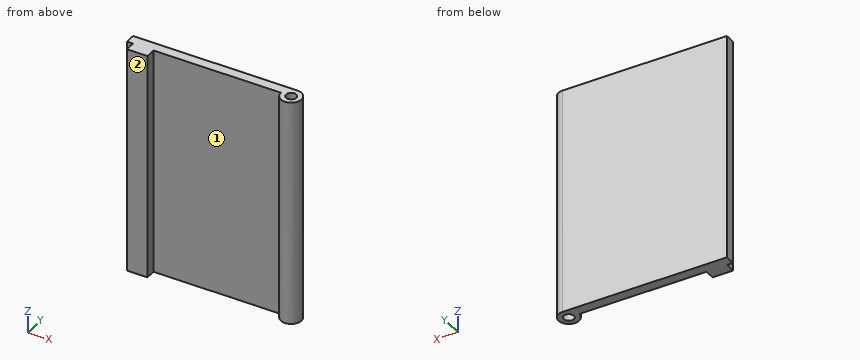
from build123d import *

# Parameters (mm, degrees)
F0_W     = 80
F0_H     = 110
F1_DEPTH = 5
F2_R     = 5
F2_W     = 10
F2_H     = 5
F3_DEPTH = 110
F4_R     = 2.5
F5_DEPTH = 110


with BuildPart() as f1:
    # F0 (on Front) → F1 (new body)
    with BuildSketch(Plane.XZ):
        with Locations((40, 55)):
            Rectangle(F0_W, F0_H)
    extrude(amount=F1_DEPTH)

    # F2 (on face) → F3 (join, through all)
    with BuildSketch(Plane.XY.offset(110)):
        with Locations((80, -5)):
            Circle(F2_R)
        with Locations((8, -7.5)):
            Rectangle(F2_W, F2_H)
    extrude(amount=-F3_DEPTH)

    # F4 (on face) → F5 (cut, through all)
    with BuildSketch(Plane.XY.offset(110)):
        with Locations((80, -5)):
            Circle(F4_R)
    extrude(amount=-F5_DEPTH, mode=Mode.SUBTRACT)


solid = f1.part
Part model, mm, in its own coordinate system. Face numbers are marked on the shaded views. A direction names the side the tool comes from. Coordinates: 2 decimals unless noted, no trailing zeros. Order: outer loops, then holes, each group sorted by start corner. A loop starts at its lowest first (then second) coordinate and runs counter-clockwise, first axis right, second up.
(1) Probe L1, parallel to Y at x = 80, z = 72.5; L2, parallel to X at y = -7, z = 47.5; L3, parallel to X at y = -6.25, z = 85. List the from-to ranges inside material, lowest first.
Check sheet entries:
L1: y = -10 to -7.5, -2.5 to 0
L2: x = 3 to 13, 75.42 to 78.5, 81.5 to 84.58
L3: x = 3 to 13, 75.16 to 77.83, 82.17 to 84.84
(2) Tool access for the marked faces 1 and 2: list every direction of +Z, -Z, +X, -X, +Y, -Y with a clear straight run to the whole face (end or side of a thin tool).
Check sheet entries:
face 1: +Z, -Z, -Y
face 2: +Z, -Z, +X, -X, -Y
(3) Pin check, flat tips, straight feed: pin 1 Ø12 at (x, z) = (70.5, 76) entering from -Y; pin 2 Ø4 at (x, z) = (34.5, 73.5) entering from +Y; pin 3 Ø3 at (x, y) = (80, -5) entering from +Z; pin 4 Ø1.5 at (y, z) = (-7.5, 81.5) entering from +X. Stop position of each tip, or through.
Check sheet entries:
pin 1: stops at y = -8.57
pin 2: stops at y = 0
pin 3: passes through
pin 4: stops at x = 84.68
(4) Slice it at A-A, the plane z = 65. Write the cut outline in (x, y).
Check sheet entries:
outline: (0, -5) - (3, -5) - (3, -10) - (13, -10) - (13, -5) - (75, -5) arc R5 ccw (long way) to (80, 0) - (0, 0) - close; hole circle Ø5 at (80, -5)
(5) Slice it at B-B, the plane x = 33.5. Write the cut outline in (y, z).
Check sheet entries:
outline: (-5, 0) - (0, 0) - (0, 110) - (-5, 110) - close
